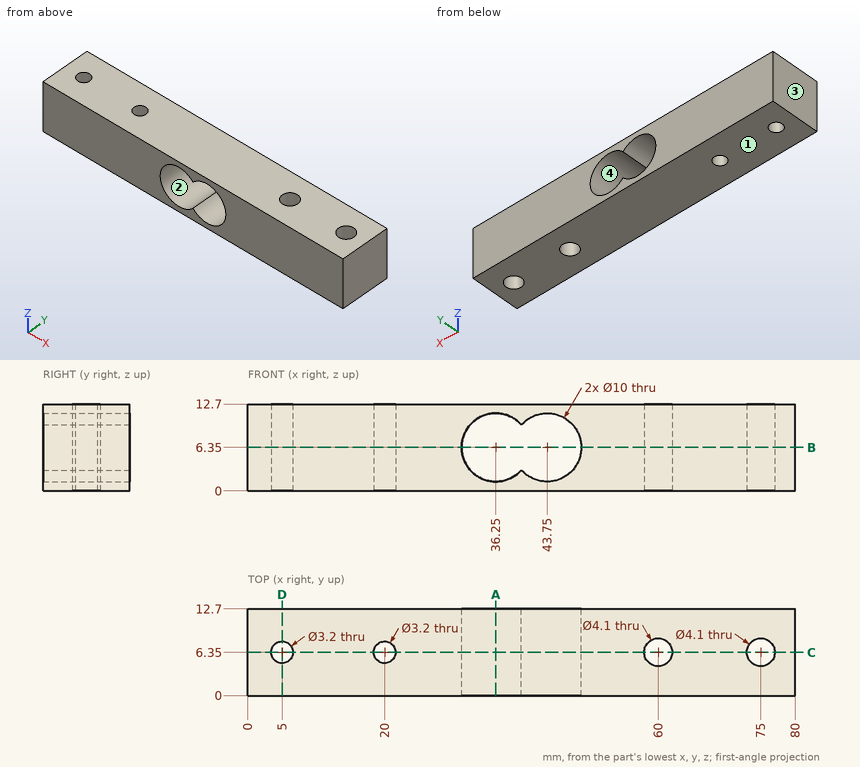
Here's the drawing with two shaded views (mm, measured from the low corner). I have some questions. Give positions to 0.01 mm unless a question says otherwise; leave off trailing zeros. Write each loop counter-clockwise with the first axis right and the second up, starting at its lowest first coordinate (ties: lowest second). Pieces come first, ordered by that corner, then holes. Notation, with made-up numbers: (-38, 16) - (6, 16) arc R14 ccw to (6, 33) - close; hole circle Ø8 at (18, 2.5). An arc over 180 degrees is marked (long way). One line per item, written item: value. Start each with the question number.
Item 1: Imagine slicing it at D-D, the plane x = 5. List the corners of the cut face in (y, z) for me.
Item 2: Please list where these lines run through material, in increasing order: line 1 (X direction, y = 6.25, z = 6); line 2 (X direction, y = 3.5, z = 6.5); line 3 (Z direction, x = 43.75, y = 8.5). Write a range as from..to.
Item 3: Imagine slicing it at C-C, the plane y = 6.35. List the corners of the cut face in (x, z) for me, and give its area (3 significant figures).
Item 4: If we mould it in two halves opening along Z, with no side actions, what happens to the marked faces 1, 2, 3 and 4? For each: +Z half, -Z half, draft (parallel to the pull), parting line (faces both ways), or undercut.
Item 5: Imagine slicing it at A-A, the plane x = 36.25. List the corners of the cut face in (y, z) for me, and give its area (3 significant figures).
Item 6: Imagine slicing it at B-B, the plane z = 6.35. List the corners of the cut face in (x, y) for me, and give its area (3 significant figures).
Geometry says:
1. outline: (0, 0) - (4.75, 0) - (4.75, 12.7) - (0, 12.7) - close; (7.95, 0) - (12.7, 0) - (12.7, 12.7) - (7.95, 12.7) - close
2. line 1: 0..3.4, 6.6..18.4, 21.6..31.26, 48.74..57.95, 62.05..72.95, 77.05..80
2. line 2: 0..31.25, 48.75..80
2. line 3: 0..1.35, 11.35..12.7
3. outline: (0, 0) - (3.4, 0) - (3.4, 12.7) - (0, 12.7) - close; (6.6, 0) - (18.4, 0) - (18.4, 12.7) - (6.6, 12.7) - close; (21.6, 0) - (57.95, 0) - (57.95, 12.7) - (21.6, 12.7) - close; (62.05, 0) - (72.95, 0) - (72.95, 12.7) - (62.05, 12.7) - close; (77.05, 0) - (80, 0) - (80, 12.7) - (77.05, 12.7) - close; hole (40, 3.04) arc R5 ccw (long way) to (40, 9.66) arc R5 ccw (long way) to start
3. area: 685 mm^2
4. face 1: -Z half
4. face 2: undercut
4. face 3: draft
4. face 4: undercut
5. outline: (0, 0) - (12.7, 0) - (12.7, 1.35) - (0, 1.35) - close; (0, 11.35) - (12.7, 11.35) - (12.7, 12.7) - (0, 12.7) - close
5. area: 34.3 mm^2
6. outline: (0, 0) - (31.25, 0) - (31.25, 12.7) - (0, 12.7) - close; (48.75, 0) - (80, 0) - (80, 12.7) - (48.75, 12.7) - close; hole circle Ø3.2 at (5, 6.35); hole circle Ø3.2 at (20, 6.35); hole circle Ø4.1 at (60, 6.35); hole circle Ø4.1 at (75, 6.35)
6. area: 751 mm^2
